```python
from build123d import *

# Parameters (mm, degrees)
SKETCH1_W                  = 370
SKETCH1_H                  = 160
KICH_THUOC_TONG_QUAN_DEPTH = 1
LO_CHOT_CO_DINH_REACH      = 405.114
SKETCH2_W                  = 10
SKETCH2_H                  = 10
LO_THONG_KHI_REACH         = 405.114
SKETCH3_R                  = 5


with BuildPart() as part:
    # Sketch1 → kich_thuoc_tong_quan (new body)
    with BuildSketch(Plane.XY):
        with Locations((185, 80)):
            Rectangle(SKETCH1_W, SKETCH1_H)
    extrude(amount=KICH_THUOC_TONG_QUAN_DEPTH)

    # Sketch2 → lo_chot_co_dinh (cut, up to next)
    with BuildSketch(Plane.XY.offset(1), mode=Mode.PRIVATE) as lo_chot_co_dinh_sk1:
        with Locations((5, 145)):
            Rectangle(SKETCH2_W, SKETCH2_H)
    lo_chot_co_dinh_tool1 = extrude(lo_chot_co_dinh_sk1.sketch, amount=-LO_CHOT_CO_DINH_REACH, mode=Mode.PRIVATE) & part.part
    # Sketch2 → lo_chot_co_dinh (cut, up to next)
    with BuildSketch(Plane.XY.offset(1), mode=Mode.PRIVATE) as lo_chot_co_dinh_sk2:
        with Locations((365, 145)):
            Rectangle(SKETCH2_W, SKETCH2_H)
    lo_chot_co_dinh_tool2 = extrude(lo_chot_co_dinh_sk2.sketch, amount=-LO_CHOT_CO_DINH_REACH, mode=Mode.PRIVATE) & part.part
    # Sketch2 → lo_chot_co_dinh (cut, up to next)
    with BuildSketch(Plane.XY.offset(1), mode=Mode.PRIVATE) as lo_chot_co_dinh_sk3:
        with Locations((365, 15)):
            Rectangle(SKETCH2_W, SKETCH2_H)
    lo_chot_co_dinh_tool3 = extrude(lo_chot_co_dinh_sk3.sketch, amount=-LO_CHOT_CO_DINH_REACH, mode=Mode.PRIVATE) & part.part
    # Sketch2 → lo_chot_co_dinh (cut, up to next)
    with BuildSketch(Plane.XY.offset(1), mode=Mode.PRIVATE) as lo_chot_co_dinh_sk4:
        with Locations((5, 15)):
            Rectangle(SKETCH2_W, SKETCH2_H)
    lo_chot_co_dinh_tool4 = extrude(lo_chot_co_dinh_sk4.sketch, amount=-LO_CHOT_CO_DINH_REACH, mode=Mode.PRIVATE) & part.part
    add(lo_chot_co_dinh_tool1.solids().sort_by_distance((5, 145, 1))[0], mode=Mode.SUBTRACT)
    add(lo_chot_co_dinh_tool2.solids().sort_by_distance((365, 145, 1))[0], mode=Mode.SUBTRACT)
    add(lo_chot_co_dinh_tool3.solids().sort_by_distance((365, 15, 1))[0], mode=Mode.SUBTRACT)
    add(lo_chot_co_dinh_tool4.solids().sort_by_distance((5, 15, 1))[0], mode=Mode.SUBTRACT)

    # Sketch3 → lo_thong_khi (cut, up to next)
    with BuildSketch(Plane.XY.offset(1), mode=Mode.PRIVATE) as lo_thong_khi_sk1:
        with Locations((340, 110)):
            Circle(SKETCH3_R)
    lo_thong_khi_tool1 = extrude(lo_thong_khi_sk1.sketch, amount=-LO_THONG_KHI_REACH, mode=Mode.PRIVATE) & part.part
    # Sketch3 → lo_thong_khi (cut, up to next)
    with BuildSketch(Plane.XY.offset(1), mode=Mode.PRIVATE) as lo_thong_khi_sk2:
        with Locations((340, 50)):
            Circle(SKETCH3_R)
    lo_thong_khi_tool2 = extrude(lo_thong_khi_sk2.sketch, amount=-LO_THONG_KHI_REACH, mode=Mode.PRIVATE) & part.part
    add(lo_thong_khi_tool1.solids().sort_by_distance((340, 110, 1))[0], mode=Mode.SUBTRACT)
    add(lo_thong_khi_tool2.solids().sort_by_distance((340, 50, 1))[0], mode=Mode.SUBTRACT)


solid = part.part
```
Here's how the part is built. I have some questions about the finished solid (model axes, mm). Give positions to 0.01 mm unless a question says otherwise; leave off trailing zeros. Order: outer loops, then holes, each group sorted by start corner. A loop starts at its lowest first (then second) coordinate and runs counter-clockwise, first axis right, second up. Notation, with made-up numbers: M 26.5,14 L 69.5,14 A20 ccw 69.5,23 Z; hole C 58,72.25 d11. An arc over 180 degrees is marked long. Use a Markdown table: item, result. Add a question column.
1. I need wall thicknesses on probe 1 along Y at (x, z) = (340, 0.4); probe 2 along X at (y, z) = (14, 0.3); probe 3 along X at (y, z) = (106, 0.45). Which ranges of each line are inside material? Lowest first, please. Write a range as from..to.
2. Suppose I cut it at A-A (y = 50). List the corners of the cut face in (x, z) for me, and give its area (3 significant figures).
3. Suppose I cut it at B-B (x = 340). List the corners of the cut face in (y, z) for me.
4. If we mould it in two halves opening along X, with no side actions, what happens to faces 1 (the flat face through (182, 81, 1)), 2 (the cylindrical face through (344.77, 51.5, 0.51))? For each: +X half, -X half, draft (parallel to the pull), parting line (faces both ways), or undercut.
Results list:
| question | item | result |
|---|---|---|
| 1 | probe 1 | y = 0..45, 55..105, 115..160 |
| 1 | probe 2 | x = 10..360 |
| 1 | probe 3 | x = 0..337, 343..370 |
| 2 | outline | M 0,0 L 335,0 L 335,1 L 0,1 Z; M 345,0 L 370,0 L 370,1 L 345,1 Z |
| 2 | area | 360 mm² |
| 3 | outline | M 0,0 L 45,0 L 45,1 L 0,1 Z; M 55,0 L 105,0 L 105,1 L 55,1 Z; M 115,0 L 160,0 L 160,1 L 115,1 Z |
| 4 | face 1 | draft |
| 4 | face 2 | undercut |
